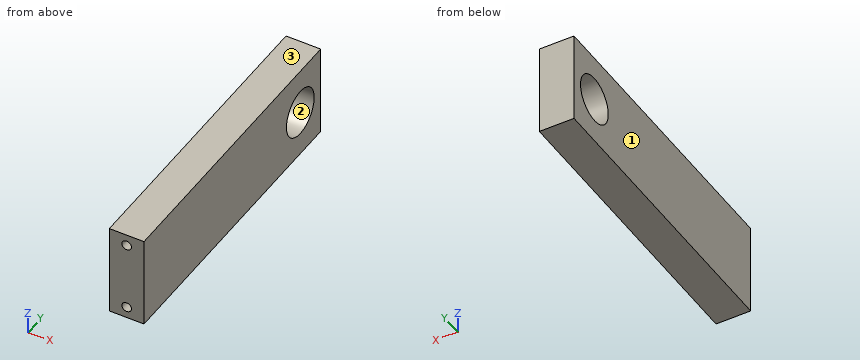
Autodesk Inventor part; units mm, degrees
ref_plane "YZ Plane" through (0, 0, 0) normal (1, 0, 0) x (0, 1, 0)
ref_plane "XZ Plane" through (0, 0, 0) normal (0, 1, 0) x (-1, 0, 0)
ref_plane "XY Plane" through (0, 0, 0) normal (0, 0, 1) x (1, 0, 0)
sketch "Sketch1" plane through (0, 0, 0) normal (1, 0, 0) x (0, 1, 0)
  line L0 (0, 0) -> (82.55, 0)
  line L1 (82.55, 0) -> (82.55, -25.4)
  line L2 (82.55, -25.4) -> (0, -25.4)
  line L3 (0, -25.4) -> (0, 0)
  circle A0 centre (73.025, -12.7) radius 6.477
  dimension "d0" = 82.55
  dimension "d1" = 25.4
  dimension "d2" = 12.954
  dimension "d3" = 73.025
extrude "Extrusion1" add sketch "Sketch1" along normal blind 9.525
sketch "Sketch2" plane through (0, 0, -25.4) normal (0, -1, 0) x (1, 0, 0)
  line L0 (0, 0) -> (0, 25.4)
  line L1 (0, 0) -> (9.525, 0)
  line L2 (9.525, 25.4) -> (9.525, 0)
  line L3 (0, 25.4) -> (9.525, 25.4)
  point P0 (4.7625, 22.225)
  point P1 (4.7625, 3.175)
  dimension "d6" = 25.4
  dimension "d7" = 3.175
  dimension "d8" = 3.175
hole "Hole1" at (4.7625, 0, -3.175) at (4.7625, 0, -22.225) direction (0, 1, 0) diameter 2.6416 depth 25.4 tip angle 118
properties part number "SlidesPivotBracket"
Part model, mm, in its own coordinate system. Face numbers are marked on the shaded views. Coordinates: 2 decimals unless noted, no trailing zeros. Order: outer loops, then holes, each group sorted by start corner. A loop starts at its lowest first (then second) coordinate and runs counter-clockwise, first axis right, second up. Notation, with made-up numbers: (31.25, 83.25) - (87.25, 83.25) arc R12 cw to (87.25, 103.25) - close; hole circle Ø8 at (67.25, 70). An arc over 180 degrees is marked (long way). Return JSON: item names as keys, results as strings. Group by question number.
Item 1: Cut at B-B (x = 1.5). List the corners of the cut face in (y, z) (3 decimals).
Item 2: Drill centre lines: probe 1 along Y at (x, z) = (8.5, -12.5); probe 2 along Y at (x, z) = (5.5, -16.25); probe 3 along Z at (x, y) = (0.75, 69.5). Where is each one in solid material? Low to high. Write a range as from..to.
Item 3: Cut at A-A (z = -12.7). List the corners of the cut face in (x, y) (3 decimals).
Item 4: Cut at D-D (z = -9.25). List the corners of the cut face in (x, y) (3 decimals), plus the area to 3 significant figures.
Item 5: Cut at C-C (y = 9.5). List the corners of the cut face in (x, z) (1 decimal).
Item 6: Pull direction Z, two halves, no side cores. Call the marked faces 1, 2 and 3: pulls with the +Z half, pulls with the -Z half, needs draft (parallel to the pull), parting line crosses it, or undercut.
Check values:
{
 "1": {"outline": "(0, -25.4) - (82.55, -25.4) - (82.55, 0) - (0, 0) - close; hole circle Ø12.954 at (73.025, -12.7)"},
 "2": {"probe 1": "y = 0..66.55, 79.5..82.55", "probe 2": "y = 0..67.61, 78.44..82.55", "probe 3": "z = -25.4..-18.13, -7.27..0"},
 "3": {"outline": "(0, 0) - (9.525, 0) - (9.525, 66.548) - (0, 66.548) - close; (0, 79.502) - (9.525, 79.502) - (9.525, 82.55) - (0, 82.55) - close"},
 "4": {"outline": "(0, 0) - (9.525, 0) - (9.525, 67.543) - (0, 67.543) - close; (0, 78.507) - (9.525, 78.507) - (9.525, 82.55) - (0, 82.55) - close", "area": "682 mm2"},
 "5": {"outline": "(0, -25.4) - (9.5, -25.4) - (9.5, 0) - (0, 0) - close; hole circle Ø2.6 at (4.8, -22.2); hole circle Ø2.6 at (4.8, -3.2)"},
 "6": {"face 1": "needs draft", "face 2": "undercut", "face 3": "pulls with the +Z half"}
}
